Here's the drawing with two shaded views (mm, measured from the low corner). I have some questions. A direction names the side the tool comes from. Coordinates: 2 decimals unless noted, no trailing zeros. Write each loop counter-clockwise with the first axis right and the second up, starting at its lowest first coordinate (ties: lowest second). Pieces come first, ordered by that corner, then holes.
Item 1: If I drill on line 1 (Y direction, x = 8, z = 2); line 2 (Y direction, x = 17.25, z = 1.1); line 3 (X direction, y = 3, z = 4.3), over which ranges is the centre line in solid material (lowest first)?
Item 2: If we section it at D-D (x = 10.5): Please give me the cut outline in (y, z).
Item 3: If we section it at A-A (x = 5.25): Please give me the cut outline in (y, z).
Item 4: We'd pull the mould along Y, two halves only. Please class the marked faces 1, 2, 3 and 4: +Y half, -Y half, draft (parallel to the pull), parting line (faces both ways), or undercut.
Item 5: For the marked faces 5, 6, 7, 8 and 9, which set-ups out of +Z, -Z, +X, -X, +Y, -Y let a thin tool reach every point of the face, with its end or its side?
Item 6: If we section it at B-B (y = 31): Please give me the cut outline in (x, z).
Item 7: I'm going to push flat-ended pins straight in: pin 1 Ø3 at (x, y) = (9.5, 23.5) entering from +Z; pin 2 Ø2.5 at (x, z) = (11, 3.5) entering from -Y; pin 3 Ø1.5 at (y, z) = (20.5, 1.5) entering from +X; pin 4 Ø0.8 at (y, z) = (0, 2) entering from -X. Where does each tip first touch, or does it pass through?
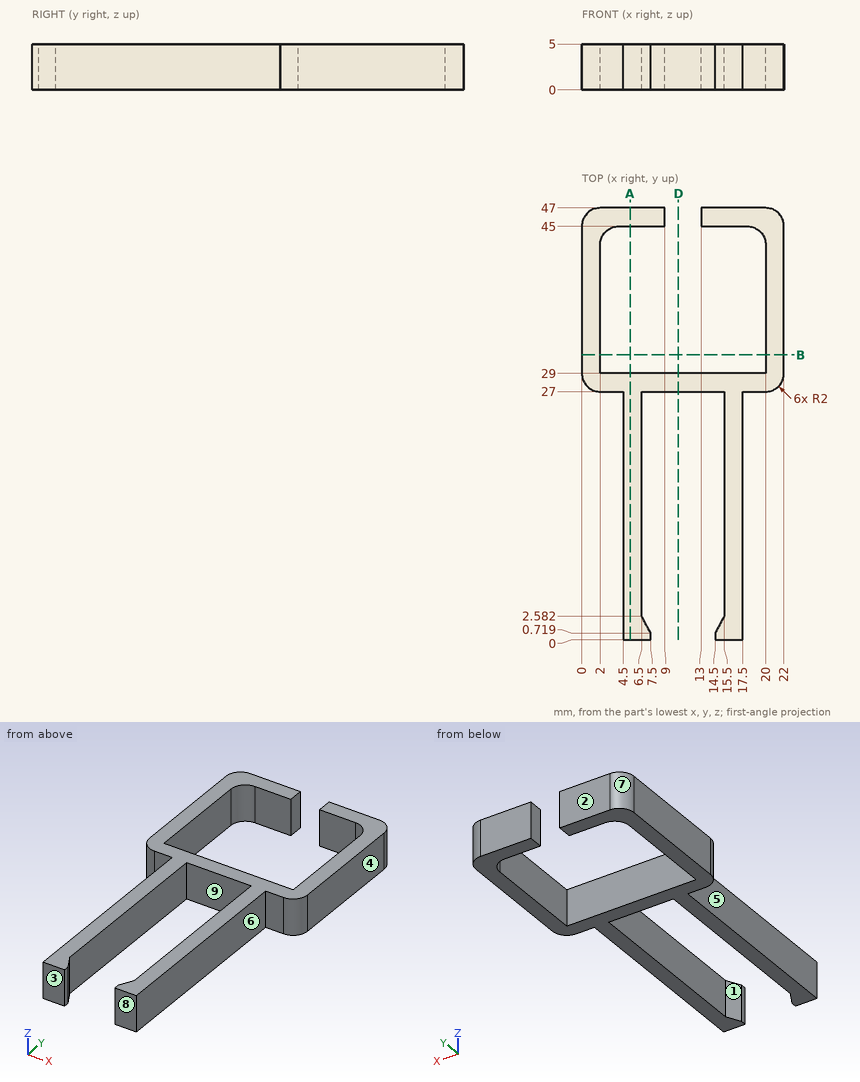
Answer list:
1. line 1: y = 27 to 29, 45 to 47
1. line 2: y = 0 to 29, 45 to 47
1. line 3: x = 4.5 to 6.5, 15.5 to 17.5
2. outline: (27, 0) - (29, 0) - (29, 5) - (27, 5) - close
3. outline: (0, 0) - (29, 0) - (29, 5) - (0, 5) - close; (45, 0) - (47, 0) - (47, 5) - (45, 5) - close
4. face 1: undercut
4. face 2: +Y half
4. face 3: -Y half
4. face 4: draft
5. face 5: +Z, -Z, -X, -Y
5. face 6: +Z, -Z, +X, -Y
5. face 7: +Z, -Z, -X, +Y
5. face 8: +Z, -Z, +X, -X, -Y
5. face 9: +Z, -Z
6. outline: (0, 0) - (2, 0) - (2, 5) - (0, 5) - close; (20, 0) - (22, 0) - (22, 5) - (20, 5) - close
7. pin 1: passes through
7. pin 2: stops at y = 27
7. pin 3: stops at x = 17.5
7. pin 4: stops at x = 4.5
